Solid Edge part; units mm, degrees
sketch "Sketch1" plane through (0, 0, 0) normal (0, 0, 1) x (1, 0, 0)
  line L0 (-21.209, -21.209) -> (21.209, -21.209)
  line L1 (21.209, -21.209) -> (21.209, 21.209)
  line L2 (21.209, 21.209) -> (-21.209, 21.209)
  line L3 (-21.209, 21.209) -> (-21.209, -21.209)
  dimension "D1" = 21.209
  dimension "D2" = 21.209
extrude "Protrusion1" add sketch "Sketch1" along normal blind 46.99
hole "Hole_1" at (-15.494, -15.494, 46.99) direction (0, 0, -1) diameter 2.459 depth 5.16 tip angle 118
hole "Hole1" at (15.494, -15.494, 46.99) direction (0, 0, -1) diameter 2.459 depth 5.16 tip angle 118
hole "Hole2" at (15.494, 15.494, 46.99) direction (0, 0, -1) diameter 2.459 depth 5.16 tip angle 118
hole "Hole3" at (-15.494, 15.494, 46.99) direction (0, 0, -1) diameter 2.459 depth 5.16 tip angle 118
sketch "Sketch2" plane through (0, 0, 46.99) normal (0, 0, 1) x (0, -1, 0)
  circle A0 centre (0, 0) radius 14.2875
extrude "CircleIndent" cut sketch "Sketch2" against normal blind 0.508
sketch "Sketch3" plane through (0, 0, 46.482) normal (0, 0, 1) x (0, -1, 0)
  circle A0 centre (0, 0) radius 11.0109
extrude "CenteringCircle" add sketch "Sketch3" along normal blind 2.794
sketch "Sketch4" plane through (0, 0, 49.276) normal (0, 0, 1) x (0, -1, 0)
  circle A0 centre (0, 0) radius 4.5974
extrude "ShaftHole" cut sketch "Sketch4" against normal blind 3.556
chamfer "SideChamfer" distance 4.4136 angle 45 4 edges at (21.209, -21.209, 23.495) (-21.209, -21.209, 23.495) (21.209, 21.209, 23.495) (-21.209, 21.209, 23.495)
sketch "Sketch5" plane through (19.0022, -19.0022, 23.495) normal (0.7071, -0.7071, 0) x (0, 0, -1)
  line L0 (-11.684, -13.6206) -> (9.9845, -13.6206)
  line L1 (9.9845, -13.6206) -> (9.9845, 11.7794)
  line L2 (9.9845, 11.7794) -> (-11.684, 11.7794)
  line L3 (-11.684, 11.7794) -> (-11.684, -13.6206)
extrude "SideCutout" cut sketch "Sketch5" against normal blind 2.0828
mirror "Mirror1" about plane through (0, 0, 0) normal (1, 0, 0) of "SideCutout"
mirror "Mirror2" about plane through (0, 0, 0) normal (0, -1, 0) of "SideCutout", "Mirror1"
properties material "Steel"
Geometry: final body of the model. Coordinates: model frame, mm. A direction names the side the tool comes from. Round coordinates to 2 decimals unless told otherwise and drop trailing zeros. Order: outer loops, then holes, each group sorted by start corner. A loop starts at its lowest first (then second) coordinate and runs counter-clockwise, first axis right, second up.
Q1. Material intervals for probe 1 along X at (y, z) = (0, 48.1); probe 2 along Z at (x, y) = (14, 11.5); probe 3 along Z at (x, y) = (13.5, -3), sorted ascending.
Result sheet:
probe 1: x = -11.01 to -4.6, 4.6 to 11.01
probe 2: z = 0 to 46.99
probe 3: z = 0 to 46.48
Q2. Section D-D, the plane z = 26. Output: boundary loops of the cut face in (x, y).
Result sheet:
outline: (-21.21, -13.85) - (-13.85, -21.21) - (13.85, -21.21) - (21.21, -13.85) - (21.21, 13.85) - (13.85, 21.21) - (-13.85, 21.21) - (-21.21, 13.85) - close
Q3. Section B-B, the plane y = 0. Output: boundary loops of the cut face in (x, z), and give its area (3 significant figures).
Result sheet:
outline: (-21.21, 0) - (21.21, 0) - (21.21, 46.99) - (14.29, 46.99) - (14.29, 46.48) - (11.01, 46.48) - (11.01, 49.28) - (4.6, 49.28) - (4.6, 45.72) - (-4.6, 45.72) - (-4.6, 49.28) - (-11.01, 49.28) - (-11.01, 46.48) - (-14.29, 46.48) - (-14.29, 46.99) - (-21.21, 46.99) - close
area: 2,010 mm2
Q4. Section A-A, the plane z = 7. Output: boundary loops of the cut face in (x, y), and give its area (3 significant figures).
Result sheet:
outline: (-21.21, -16.8) - (-16.8, -21.21) - (16.8, -21.21) - (21.21, -16.8) - (21.21, 16.8) - (16.8, 21.21) - (-16.8, 21.21) - (-21.21, 16.8) - close
area: 1,760 mm2
Q5. Pin query (flat end, axial travel): pin 1 (8 mm diameter, centred on x = 18.5, y = -16.5, fed in from +Z); pin 2 (2 mm diameter, centred on x = 15.494, y = 15.494, fed in from +Z); pin 3 (3 mm diameter, centred on x = 0, y = 1, fed in from +Z). Return the tip coordinate at first contact, or that it passes through.
Result sheet:
pin 1: stops at z = 46.99
pin 2: stops at z = 41.69
pin 3: stops at z = 45.72
Q6. Access query for faces 1 (the face through (18, 18, 35.179)), 2 (the face through (21.209, 0, 23)), 3 (the face through (-18.971, 19.033, 41.002)), 4 (the face through (-17.58, -17.48, 24.5)), 5 (the face through (0, 0, 45.72)). Directions: +Z, -Z, +X, -X, +Y, -Y. A direction counts if a zero-diameter tool reaches every point of the face in a straight line with its end or side. Return the directions, or none.
Result sheet:
face 1: +X, +Y
face 2: +Z, -Z, +X, +Y, -Y
face 3: +Z, -Z, -X, +Y
face 4: -X, -Y
face 5: +Z
Q7. Mould query, pull axis Y, two halves, no side actions, for faces 6 (the face through (17.48, -17.58, 24.5)), 7 (the face through (-18, 18, 35.179)), 8 (the face through (-1.761, -4.247, 47.523)). Classes: released by +Y, released by -Y, zero draft, split by the parting line, or undercut.
Result sheet:
face 6: released by -Y
face 7: zero draft
face 8: undercut
